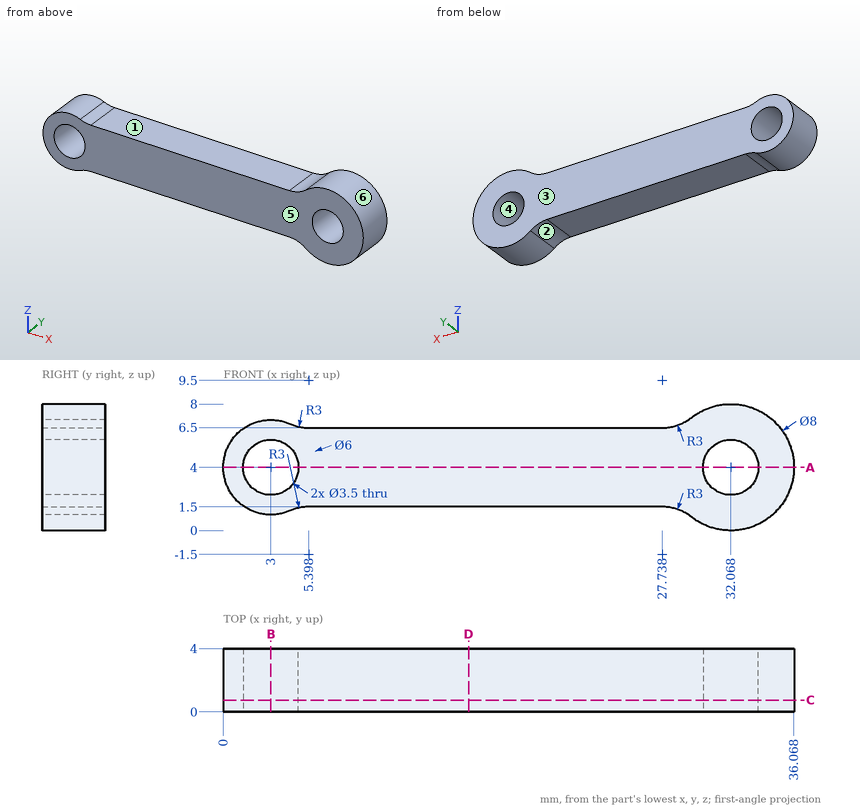
Study the drawing (mm; zero at the part's minimum x, y, z) and answer. A direction names the side the tool comes from. Give positions to 0.01 mm unless a question says otherwise; leave off trailing zeros. Write each loop counter-clockwise with the first axis right and the second up, starting at its lowest first coordinate (ties: lowest second). Pieces come first, ordered by that corner, then holes. Notation, with made-up numbers: (88.5, -2.75) -> (111.5, -2.75) arc R8 cw to (111.5, 9.25) -> close; hole circle Ø10 at (28.25, 58). An arc over 180 degrees is marked (long way). Answer in a Markdown table with one row per item.
1) Section A-A on z = 4 is taken. Give the vertices of the cut face in (x, y).
Results list:
| item | result |
|---|---|
| outline | (0, 0) -> (1.25, 0) -> (1.25, 4) -> (0, 4) -> close; (4.75, 0) -> (30.32, 0) -> (30.32, 4) -> (4.75, 4) -> close; (33.82, 0) -> (36.07, 0) -> (36.07, 4) -> (33.82, 4) -> close |
2) Determine the mould class of the marked faces 4, 5 and 6 for opening direction X: released by +X, released by -X, zero draft, split by the parting line, or undercut.
Results list:
| item | result |
|---|---|
| face 4 | undercut |
| face 5 | zero draft |
| face 6 | split by the parting line |
3) Section C-C on y = 0.75 is taken. Give the vertices of the cut face in (x, z).
Results list:
| item | result |
|---|---|
| outline | (4.2, 1.25) arc R3 cw to (5.4, 1.5) -> (27.74, 1.5) arc R3 cw to (29.59, 0.86) arc R4 ccw (long way) to (29.59, 7.14) arc R3 cw to (27.74, 6.5) -> (5.4, 6.5) arc R3 cw to (4.2, 6.75) arc R3 ccw (long way) to start; hole circle Ø3.5 at (3, 4); hole circle Ø3.5 at (32.07, 4) |
4) Straight lines are drawn through the part: line 1 (Z direction, x = 3, y = 2.2); line 2 (Z direction, x = 24, y = 0.45); line 3 (X direction, y = 1.15, z = 0.5) (1 decimal). For each, find the intervals that lie inside material, in ascending order. Write a range as [from, to].
Results list:
| item | result |
|---|---|
| line 1 | [1, 2.25], [5.75, 7] |
| line 2 | [1.5, 6.5] |
| line 3 | [30.1, 34] |
5) Each of these flat-tipped pins is pushed along its axis until it touches: pin 1 Ø1 at (y, z) = (1.5, 3) entering from -X; pin 2 Ø4.5 at (x, z) = (3, 4) entering from -Y. Where does it stop, or does it pass through?
Results list:
| item | result |
|---|---|
| pin 1 | x = 0.04 |
| pin 2 | y = 0 |
6) Section D-D on x = 15.5 is taken. Give the vertices of the cut face in (y, z), plus the area to 3 significant figures.
Results list:
| item | result |
|---|---|
| outline | (0, 1.5) -> (4, 1.5) -> (4, 6.5) -> (0, 6.5) -> close |
| area | 20.0 mm^2 |
7) Section B-B on x = 3 is taken. Give the vertices of the cut face in (y, z), plus the area to 3 significant figures.
Results list:
| item | result |
|---|---|
| outline | (0, 1) -> (4, 1) -> (4, 2.25) -> (0, 2.25) -> close; (0, 5.75) -> (4, 5.75) -> (4, 7) -> (0, 7) -> close |
| area | 10.0 mm^2 |
8) A tool of negligible diameter and unlimited length cuts with its end or side. For the marked faces 1, 2 and 3, from which of +Z, -Z, +X, -X, +Y, -Y can it reach the whole face along a straight path? Write none if from no direction.
Results list:
| item | result |
|---|---|
| face 1 | +Z, +Y, -Y |
| face 2 | -Z, +Y, -Y |
| face 3 | +Z, -Z, +X, -X, +Y |
